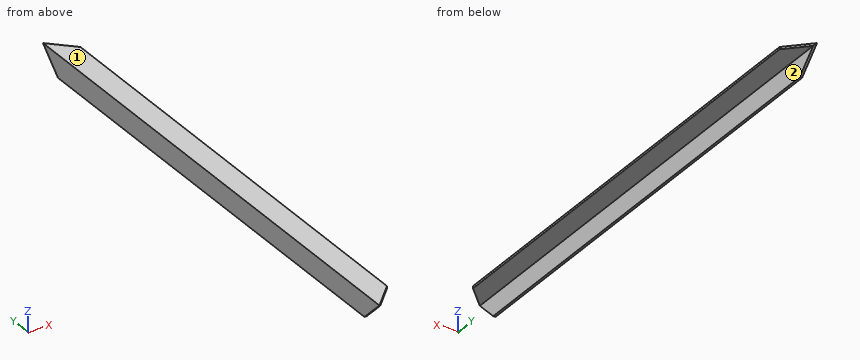
```python
from build123d import *

# Parameters (mm, degrees)
F1_DEPTH = 450
F3_DEPTH = 40
F5_DEPTH = 40


with BuildPart() as f1:
    # F0 (on Front) → F1 (new body, symmetric)
    with BuildSketch(Plane.XZ):
        Polygon((0, 40), (0, 0), (4, 0), (4, 36), (40, 36), (40, 40), align=None)
    extrude(amount=F1_DEPTH, both=True)

    # F2 (on face) → F3 (cut)
    with BuildSketch(Plane(origin=(0, 0, 0), x_dir=(0, -1, 0), z_dir=(-1, 0, 0))):
        Polygon((-410, 0), (-450, 40), (-450, 0), align=None)
        Polygon((450, 0), (450, 40), (410, 0), align=None)
    extrude(amount=-F3_DEPTH, mode=Mode.SUBTRACT)

    # F4 (on face) → F5 (cut)
    with BuildSketch(Plane.XY.offset(40)):
        Polygon((40, 450), (0, 450), (40, 410), align=None)
        Polygon((40, -410), (0, -450), (40, -450), align=None)
    extrude(amount=-F5_DEPTH, mode=Mode.SUBTRACT)


solid = f1.part
```
Model file for the job. Use its own axes, mm. Face numbers are marked on the shaded views. A direction names the side the tool comes from. Coordinates: 2 decimals unless noted, no trailing zeros. Order: outer loops, then holes, each group sorted by start corner. A loop starts at its lowest first (then second) coordinate and runs counter-clockwise, first axis right, second up. Notation, with made-up numbers: (63, -28.75) -> (107, -28.75) arc R26 cw to (107, 10.25) -> close; hole circle Ø4 at (-4.5, 79). An arc over 180 degrees is marked (long way). Answer as a JSON object with one key per item and string values. Group by question number.
1) Flat gauge pins, fed straight in: pin 1 (1.5 mm diameter, centred on x = 17, y = 358.5, fed in from -Z); pin 2 (3 mm diameter, centred on y = 56, z = 27.5, fed in from +X). Where does each tip first touch, or does it go through?
2) Cut at B-B, the plane y = -46. Write the cut outline in (x, z), then the cut area to 3 significant figures.
3) Which spindle directions (+Z, -Z, +X, -X, +Y, -Y) get a long thin tool onto all of the face, cutting with end or side? Do the marked faces 1 and 2. Say none if no direction does.
4) Drill centre lines: L1, parallel to X at y = -31.5, z = 20; L2, parallel to Z at x = 6, y = -166; L3, parallel to Y at x = 2, z = 38.5. Where is each one in solid material? Low to high.
5) Cut at C-C, the plane z = 9. Write the cut outline in (x, y).
6) Cut at A-A, the plane x = 21. Write the cut outline in (y, z), then the cut area to 3 significant figures.
Check values:
{
 "1": {"pin 1": "stops at z = 36", "pin 2": "stops at x = 4"},
 "2": {"outline": "(0, 0) -> (4, 0) -> (4, 36) -> (40, 36) -> (40, 40) -> (0, 40) -> close", "area": "304 mm²"},
 "3": {"face 1": "+Z, +X, -X, +Y, -Y", "face 2": "-Z, +X, +Y, -Y"},
 "4": {"L1": "x = 0 to 4", "L2": "z = 36 to 40", "L3": "y = -448 to 448"},
 "5": {"outline": "(0, -419) -> (4, -419) -> (4, 419) -> (0, 419) -> close"},
 "6": {"outline": "(-429, 36) -> (429, 36) -> (429, 40) -> (-429, 40) -> close", "area": "3,430 mm²"}
}
